Can you work these out from the model? Positions are in its coordinate system, mm. Coordinates: 2 decimals unless noted, no trailing zeros. Loops run counter-clockwise (first coordinate to the right, second up) from the corner with the lowest first, then second, coordinate; pieces in that order, holes last.
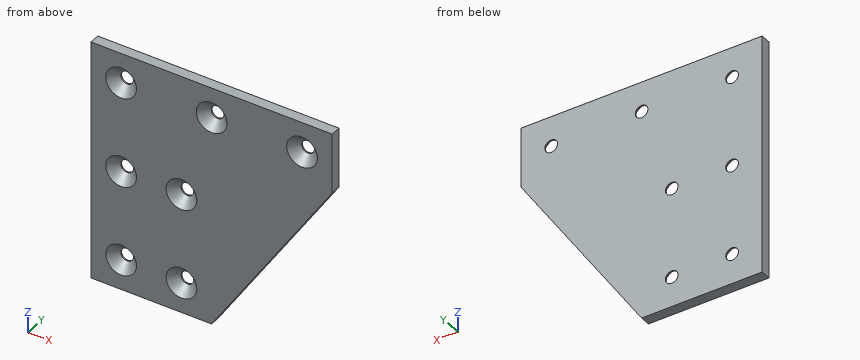
```python
from build123d import *

# Parameters (mm, degrees)
BOSS_EXTRUDE1_DEPTH = 3.416
SKETCH2_R           = 2.1
CUT_EXTRUDE1_DEPTH  = 4
CHAMFER1_SIZE       = 3


with BuildPart() as part:
    # Sketch1 → Boss-Extrude1 (new body)
    with BuildSketch(Plane(origin=(0, 0, 0), x_dir=(1, 0, 0), z_dir=(0, 1, 0))):
        Polygon((0, 0), (80, 0), (80, 20), (40, 80), (0, 80), align=None)
    extrude(amount=BOSS_EXTRUDE1_DEPTH)

    # Sketch2 → Cut-Extrude1 (cut)
    with BuildSketch(Plane(origin=(0, 3.416, 0), x_dir=(1, 0, 0), z_dir=(0, 1, 0))):
        with Locations((10, 10)):
            Circle(SKETCH2_R)
        with Locations((40, 10)):
            Circle(SKETCH2_R)
        with Locations((70, 10)):
            Circle(SKETCH2_R)
        with Locations((30, 40)):
            Circle(SKETCH2_R)
        with Locations((30, 70)):
            Circle(SKETCH2_R)
        with Locations((10, 40)):
            Circle(SKETCH2_R)
        with Locations((10, 70)):
            Circle(SKETCH2_R)
    extrude(amount=-CUT_EXTRUDE1_DEPTH, mode=Mode.SUBTRACT)

    # Chamfer1
    chamfer1_edges = [part.edges().sort_by_distance(p)[0] for p in [
        (7.9, 0, -70),
        (7.9, 0, -40),
        (27.9, 0, -70),
        (27.9, 0, -40),
        (67.9, 0, -10),
        (37.9, 0, -10),
        (7.9, 0, -10),
    ]]
    chamfer(chamfer1_edges, length=CHAMFER1_SIZE)


solid = part.part
```
Item 1: Suppose I cut it at D-D, the plane x = 10. Please give me the cut outline in (y, z), plus the area to 3 significant figures.
Results are:
outline: (0, -80) - (3.42, -80) - (3.42, -72.1) - (3, -72.1) - (0, -75.1) - close; (0, -64.9) - (3, -67.9) - (3.42, -67.9) - (3.42, -42.1) - (3, -42.1) - (0, -45.1) - close; (0, -34.9) - (3, -37.9) - (3.42, -37.9) - (3.42, -12.1) - (3, -12.1) - (0, -15.1) - close; (0, -4.9) - (3, -7.9) - (3.42, -7.9) - (3.42, 0) - (0, 0) - close
area: 203 mm2
Item 2: Suppose I cut it at A-A, the plane x = 70. Please give me the cut outline in (y, z), plus the area to 3 significant figures.
Results are:
outline: (0, -35) - (3.42, -35) - (3.42, -12.1) - (3, -12.1) - (0, -15.1) - close; (0, -4.9) - (3, -7.9) - (3.42, -7.9) - (3.42, 0) - (0, 0) - close
area: 96.2 mm2
Item 3: I'm going to push flat-ended pins straight in: P1, Ø4, axis at x = 51.5, z = -64.5, coming from the -Y side; P2, Ø5, axis at x = 30, z = -40, coming from the -Y side; P3, Ø5.5, axis at x = 10, z = -70, coming from the -Y side. Where does each tip first touch, or does it pass through?
Results are:
P1: stops at y = 0
P2: stops at y = 2.6
P3: stops at y = 2.35
Item 4: I need wall thicknesses on line 1 along X through (y, z) = (3.25, -10); line 2 along Z through (x, y) = (10, 3.1); line 3 along Z through (x, y) = (8.5, 3.15). Which ranges of each line are inside material? Lowest first, please.
Results are:
line 1: x = 0 to 7.9, 12.1 to 37.9, 42.1 to 67.9, 72.1 to 80
line 2: z = -80 to -72.1, -67.9 to -42.1, -37.9 to -12.1, -7.9 to 0
line 3: z = -80 to -71.47, -68.53 to -41.47, -38.53 to -11.47, -8.53 to 0
Item 5: Suppose I cut it at C-C, the plane z = -10. Please give me the cut outline in (x, y), plus the area to 3 significant figures.
Results are:
outline: (0, 0) - (4.9, 0) - (7.9, 3) - (7.9, 3.42) - (0, 3.42) - close; (12.1, 3) - (15.1, 0) - (34.9, 0) - (37.9, 3) - (37.9, 3.42) - (12.1, 3.42) - close; (42.1, 3) - (45.1, 0) - (64.9, 0) - (67.9, 3) - (67.9, 3.42) - (42.1, 3.42) - close; (72.1, 3) - (75.1, 0) - (80, 0) - (80, 3.42) - (72.1, 3.42) - close
area: 203 mm2
Item 6: Suppose I cut it at B-B, the plane y = 1.5. Please give me the cut outline in (x, z), plus the area to 4 significant figures.
Results are:
outline: (0, -80) - (40, -80) - (80, -20) - (80, 0) - (0, 0) - close; hole circle Ø7.2 at (10, -70); hole circle Ø7.2 at (10, -40); hole circle Ø7.2 at (10, -10); hole circle Ø7.2 at (30, -70); hole circle Ø7.2 at (30, -40); hole circle Ø7.2 at (40, -10); hole circle Ø7.2 at (70, -10)
area: 4,915 mm2
